Design review of the part built by this model. Coordinates are the model's own, in mm. A direction names the side the tool comes from. Round coordinates to 2 decimals unless told otherwise and drop trailing zeros. Loops run counter-clockwise (first coordinate to the right, second up) from the corner with the lowest first, then second, coordinate; pieces in that order, holes last. Notation, with made-up numbers: (72.5, 5) -> (87.5, 5) arc R21 cw to (87.5, 37) -> close; hole circle Ø8 at (55.25, -6). An arc over 180 degrees is marked (long way). Use a Markdown table: item, result. Add a question column.
from build123d import *

# Parameters (mm, degrees)
SKETCH1_R           = 4.025
SKETCH1_R_2         = 1.65
SKETCH1_R_3         = 3
SKETCH1_W           = 9
SKETCH1_H           = 15
BOSS_EXTRUDE1_DEPTH = 5
CUT_EXTRUDE1_DEPTH  = 186.946611569
CUT_EXTRUDE2_DEPTH  = 186.946611569


with BuildPart() as part:
    # Sketch1 → Boss-Extrude1 (new body)
    with BuildSketch(Plane.XY):
        with BuildLine():
            Line((-127.0125, 29.449853865), (38.001928415, 124.720978531))
            Line((38.001928415, 124.720978531), (36.501928415, 127.319054742))
            ThreePointArc((36.501928415, 127.319054742), (42.014428415, 128.796124665), (47.526928415, 127.319054742))
            Line((47.526928415, 127.319054742), (86.498071585, 104.819054742))
            ThreePointArc((86.498071585, 104.819054742), (90.533501662, 100.783624665), (92.010571585, 95.271124665))
            Line((92.010571585, 95.271124665), (89.010571585, 95.271124665))
            Line((89.010571585, 95.271124665), (89.010571585, -95.271124665))
            Line((89.010571585, -95.271124665), (92.010571585, -95.271124665))
            ThreePointArc((92.010571585, -95.271124665), (90.533501662, -100.783624665), (86.498071585, -104.819054742))
            Line((86.498071585, -104.819054742), (47.526928415, -127.319054742))
            ThreePointArc((47.526928415, -127.319054742), (42.014427779, -128.796124665), (36.501927313, -127.319054106))
            Line((36.501927313, -127.319054106), (38.001927613, -124.720978068))
            Line((38.001927613, -124.720978068), (-127.012489808, -29.44983436))
            Line((-127.012489808, -29.44983436), (-128.512501102, -32.047929441))
            ThreePointArc((-128.512501102, -32.047929441), (-132.547930395, -28.012499449), (-134.025, -22.5))
            Line((-134.025, -22.5), (-134.025, 22.5))
            ThreePointArc((-134.025, 22.5), (-132.547930077, 28.0125), (-128.5125, 32.047930077))
            Line((-128.5125, 32.047930077), (-127.0125, 29.449853865))
        make_face()
        with Locations((-123, 22.5)):
            Circle(SKETCH1_R, mode=Mode.SUBTRACT)
        with Locations((-123, -22.5)):
            Circle(SKETCH1_R, mode=Mode.SUBTRACT)
        with Locations((42.014428415, 117.771124665)):
            Circle(SKETCH1_R, mode=Mode.SUBTRACT)
        with Locations((80.985571585, 95.271124665)):
            Circle(SKETCH1_R, mode=Mode.SUBTRACT)
        with Locations((80.985571585, -95.271124665)):
            Circle(SKETCH1_R, mode=Mode.SUBTRACT)
        with Locations((42.014428415, -117.771124665)):
            Circle(SKETCH1_R, mode=Mode.SUBTRACT)
        with Locations((-99, 36.356406461)):
            Circle(SKETCH1_R_2, mode=Mode.SUBTRACT)
        with Locations((-99, -36.356410153)):
            Circle(SKETCH1_R_2, mode=Mode.SUBTRACT)
        with Locations((80.985571585, 67.558311744)):
            Circle(SKETCH1_R_2, mode=Mode.SUBTRACT)
        with Locations((18.014425217, 103.914720051)):
            Circle(SKETCH1_R_2, mode=Mode.SUBTRACT)
        with Locations((18.014428415, -103.914718205)):
            Circle(SKETCH1_R_2, mode=Mode.SUBTRACT)
        with Locations((80.985574783, -67.558309898)):
            Circle(SKETCH1_R_2, mode=Mode.SUBTRACT)
        with Locations((-123, 12)):
            Circle(SKETCH1_R_3, mode=Mode.SUBTRACT)
        with Locations((-123, -12)):
            Circle(SKETCH1_R_3, mode=Mode.SUBTRACT)
        with Locations((71.892304845, 100.521124665)):
            Circle(SKETCH1_R_3, mode=Mode.SUBTRACT)
        with Locations((51.107695155, 112.521124665)):
            Circle(SKETCH1_R_3, mode=Mode.SUBTRACT)
        with Locations((51.107695155, -112.521124665)):
            Circle(SKETCH1_R_3, mode=Mode.SUBTRACT)
        with Locations((71.892304845, -100.521124665)):
            Circle(SKETCH1_R_3, mode=Mode.SUBTRACT)
        Polygon((57.254809472, -114.168238983), (70.245190528, -106.668238983), (65.745190528, -98.874010348), (52.754809472, -106.374010348), align=None, mode=Mode.SUBTRACT)
        with Locations((-123, 0)):
            Rectangle(SKETCH1_W, SKETCH1_H, mode=Mode.SUBTRACT)
        Polygon((65.745190528, 98.874010348), (52.754809472, 106.374010348), (57.254809472, 114.168238983), (70.245190528, 106.668238983), align=None, mode=Mode.SUBTRACT)
    extrude(amount=BOSS_EXTRUDE1_DEPTH)

    # Sketch2 → Cut-Extrude1 (cut, through all)
    with BuildSketch(Plane.XY.offset(5)):
        Polygon((89.010571585, 1.48), (79.010571585, 1.48), (79.010571585, 3.5), (78.510571585, 3.5), (78.510571585, 2.75), (76.010571585, 2.75), (76.010571585, 1.48), (75.010571585, 1.48), (75.010571585, -1.48), (76.010571585, -1.48), (76.010571585, -2.75), (78.510571585, -2.75), (78.510571585, -3.5), (79.010571585, -3.5), (79.010571585, -1.48), (89.010571585, -1.48), align=None)
        Polygon((-43.223568195, -77.825416198), (-38.223568195, -69.16516216), (-36.474196879, -70.17516216), (-36.224196879, -69.742149458), (-36.873715932, -69.367149458), (-35.623715932, -67.202085949), (-36.723568195, -66.567085949), (-36.223568195, -65.701060545), (-38.78700339, -64.221060545), (-39.28700339, -65.087085949), (-40.386855653, -64.452085949), (-41.636855653, -66.617149458), (-42.286374706, -66.242149458), (-42.536374706, -66.67516216), (-40.78700339, -67.68516216), (-45.78700339, -76.345416198), align=None)
        Polygon((-45.78700339, 76.345416198), (-40.78700339, 67.68516216), (-42.536374706, 66.67516216), (-42.286374706, 66.242149458), (-41.636855653, 66.617149458), (-40.386855653, 64.452085949), (-39.28700339, 65.087085949), (-38.78700339, 64.221060545), (-36.223568195, 65.701060545), (-36.723568195, 66.567085949), (-35.623715932, 67.202085949), (-36.873715932, 69.367149458), (-36.224196879, 69.742149458), (-36.474196879, 70.17516216), (-38.223568195, 69.16516216), (-43.223568195, 77.825416198), align=None)
    extrude(amount=-CUT_EXTRUDE1_DEPTH, mode=Mode.SUBTRACT)

    # Sketch3 → Cut-Extrude2 (cut, through all)
    with BuildSketch(Plane.XY.offset(5)):
        Polygon((-35.672418314, -55.786425681), (-33.042712773, -67.537516271), (-25.982061715, -71.613986146), (-31.241472797, -48.111804967), align=None)
        Polygon((-26.810527281, -40.437184252), (-18.921410657, -75.690456022), (-11.8607596, -79.766925897), (-22.379581764, -32.762563537), align=None)
        Polygon((-17.226520227, -23.837201518), (-3.649426542, -84.507742511), (-0.26619791, -86.461050993), (2.041586213, -82.463852704), (-11.425936407, -22.282940485), (-15.103358833, -20.159779092), align=None)
        Polygon((-3.21460335, -27.0237571), (7.194647751, -73.538490685), (12.010892877, -65.196511647), (4.460017365, -31.454702616), align=None)
        Polygon((9.998535314, -34.652368297), (15.486616444, -59.176383442), (20.30286157, -50.834404404), (17.673156029, -39.083313814), align=None)
    extrude(amount=-CUT_EXTRUDE2_DEPTH, mode=Mode.SUBTRACT)


solid = part.part
1. Consider section A-A on y = -12. State the section outline as (x, z) points (3 decimals), plus the area to 3 significant figures.
2. For faces 4 (the face through (-132.51, -28.08, 2.46)), 5 (the face through (1.92, -49.96, 2.54)), list the 3-axis set-ups (+Z, -Z, +X, -X, +Y, -Y) from which the entire face can be reached by the end or side of a thin tool; tool diameter is ignored.
3. Consider section B-B on x = -123. State the section outline as (y, z) points (3 decimals).
4. Mouldability with a two-part tool opening along Y and no side actions: class faces 1 (the face through (67.29, -115.91, 2.46)), 2 (the face through (-86.97, 52.57, 2.46)), 3 (the face through (-22.92, -57.82, 2.54)) as +Y half, -Y half, draft (parallel to the pull), parting line (faces both ways), or undercut.
5. Consider section D-D on z = 4.2. Give the number of separate pieces and of enclosed holes in the cut face, plus the area to 3 significant figures.
6. To check wall thickness, follow probe 1 along X at (y, z) = (-6, 0.9) (3 decimals); probe 2 along X at (y, z) = (-48.5, 1.2); probe 3 along X at (y, z) = (-12.5, 3.1) (3 decimals). State the ranges of each line that lie inside material, in increasing order. Write a range as from..to.
7. Consider section C-C on x = -85.5. State the section outline as (y, z) points.
8. Insertion check: P1, Ø1.4, axis at y = 2, z = 3.5, coming from the +X side; P2, Ø0.6, axis at x = 78.5, z = 2, coming from the +Y side; P3, Ø1.5, axis at x = 90, z = 2.5, coming from the +Y side; P4, Ø3, axis at x = -99, y = -36.36, coming from the -Z side. Each pin has a flat end and moves straight along its axis. Give the tip position at first contact, or say it passes through.
Verdict:
| question | item | result |
|---|---|---|
| 1 | outline | (-134.025, 0) -> (-126, 0) -> (-126, 5) -> (-134.025, 5) -> close; (-120, 0) -> (89.011, 0) -> (89.011, 5) -> (-120, 5) -> close |
| 1 | area | 1,090 mm² |
| 2 | face 4 | +Z, -Z, -X, -Y |
| 2 | face 5 | +Z, -Z |
| 3 | outline | (-31.766, 0) -> (-26.525, 0) -> (-26.525, 5) -> (-31.766, 5) -> close; (-18.475, 0) -> (-15, 0) -> (-15, 5) -> (-18.475, 5) -> close; (-9, 0) -> (-7.5, 0) -> (-7.5, 5) -> (-9, 5) -> close; (7.5, 0) -> (9, 0) -> (9, 5) -> (7.5, 5) -> close; (15, 0) -> (18.475, 0) -> (18.475, 5) -> (15, 5) -> close; (26.525, 0) -> (31.766, 0) -> (31.766, 5) -> (26.525, 5) -> close |
| 4 | face 1 | -Y half |
| 4 | face 2 | +Y half |
| 4 | face 3 | undercut |
| 5 | separate pieces | 1 |
| 5 | enclosed holes | 26 |
| 5 | area | 35,700 mm² |
| 6 | probe 1 | x = -134.025..-127.5, -118.5..89.011 |
| 6 | probe 2 | x = -94.02..-31.47, -31.15..-25.01, -18.86..-11.71, -5.56..1.59, 8.27..13.1, 19.78..89.01 |
| 6 | probe 3 | x = -134.025..-125.958, -120.042..89.011 |
| 7 | outline | (-53.42, 0) -> (53.42, 0) -> (53.42, 5) -> (-53.42, 5) -> close |
| 8 | P1 | stops at x = 89.01 |
| 8 | P2 | stops at y = 109.61 |
| 8 | P3 | stops at y = 102.57 |
| 8 | P4 | passes through |
